Work out the finished part from the listing and answer in its coordinate system (mm). Face numbers are marked on the shaded views. A direction names the side the tool comes from. Give positions to 0.01 mm unless a question says otherwise; leave off trailing zeros. Write each loop counter-clockwise with the first axis right and the second up, starting at its lowest first coordinate (ties: lowest second). Pieces come first, ordered by that corner, then holes. Notation, with made-up numbers: (-21.75, 14.25) -> (-17.75, 14.25) arc R25 ccw to (-17.75, 48.25) -> close; hole circle Ø1 at (61, 43.5). An arc over 180 degrees is marked (long way). Write item = value, one per line. Start each with the question number.
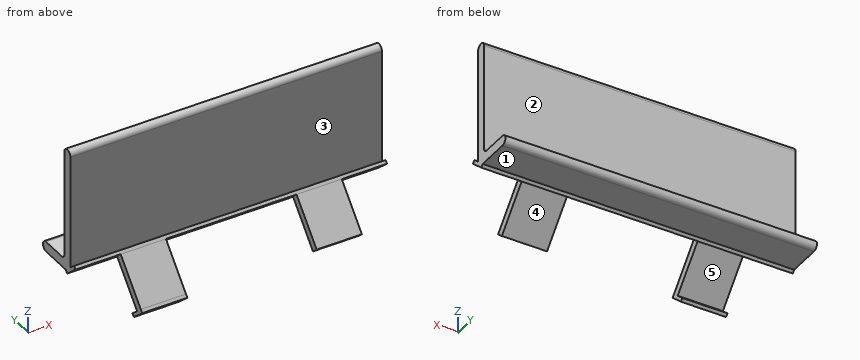
from build123d import *

# Parameters (mm, degrees)
F1_DEPTH = 155
F3_DEPTH = 155
F5_START = 22.5
F5_DEPTH = 22.5
F6_START = 110
F6_DEPTH = 22.5
F8_START = 22.5
F8_DEPTH = 22.5


# Not quite as in the source:
# - a feature of the source that left no trace in its solid (it failed there, or was rolled back) is left out


with BuildPart() as f1:
    # F0 (on Right) → F1 (new body)
    with BuildSketch(Plane.YZ):
        with BuildLine():
            Line((-25.3971134126, 39.5229434967), (-30.3971134126, 39.5229434967))
            Line((-30.3971134126, 39.5229434967), (-30.3971134126, -18.4770565033))
            ThreePointArc((-30.3971134126, -18.4770565033), (-29.811326975, -19.8912700657), (-28.3971134126, -20.4770565033))
            Line((-28.3971134126, -20.4770565033), (-10.3971134126, -20.4770565033))
            Line((-10.3971134126, -20.4770565033), (-10.3971134126, -15.4770565033))
            Line((-10.3971134126, -15.4770565033), (-23.3971134126, -15.4770565033))
            ThreePointArc((-23.3971134126, -15.4770565033), (-24.811326975, -14.8912700657), (-25.3971134126, -13.4770565033))
            Line((-25.3971134126, -13.4770565033), (-25.3971134126, 39.5229434967))
        make_face()
        with BuildLine():
            ThreePointArc((-25.3971134126, 39.5229434967), (-27.8971134126, 42.0229434967), (-30.3971134126, 39.5229434967))
            Line((-30.3971134126, 39.5229434967), (-25.3971134126, 39.5229434967))
        make_face()
        with BuildLine():
            Line((-10.3971134126, -15.4770565033), (-10.3971134126, -20.4770565033))
            ThreePointArc((-10.3971134126, -20.4770565033), (-7.8971134126, -17.9770565033), (-10.3971134126, -15.4770565033))
        make_face()
    extrude(amount=F1_DEPTH)

    # F2 (on Right) → F3 (join)
    with BuildSketch(Plane.YZ):
        Polygon((-26.6438154831, -20.4771793517), (-33.4096477321, -14.5422392527), (-34.530691973, -15.8202297886), (-27.764859724, -21.7551698876), align=None)
    extrude(amount=F3_DEPTH)

    # F4 (on Right) → F5 (join)
    with BuildSketch(Plane.YZ.offset(F5_START)):
        Polygon((-31.5236554179, -18.4579809437), (-34.530691973, -15.8202297886), (-51.0166366924, -34.614208258), (-48.0096001373, -37.2519594131), align=None)
    extrude(amount=F5_DEPTH)

    # F4 (on Right) → F6 (join)
    with BuildSketch(Plane.YZ.offset(F6_START)):
        Polygon((-31.5236554179, -18.4579809437), (-34.530691973, -15.8202297886), (-51.0166366924, -34.614208258), (-48.0096001373, -37.2519594131), align=None)
    extrude(amount=F6_DEPTH)

    # F7 (on Right) → F8 (join)
    with BuildSketch(Plane.YZ.offset(F8_START)):
        Polygon((-51.0166366924, -34.614208258), (-52.136497942, -35.8932355375), (-45.370665693, -41.8281756365), (-44.2508044434, -40.549148357), align=None)
    extrude(amount=F8_DEPTH)


solid = f1.part
(1) For the marked faces 1 and 2, determine the directions among +Z, -Z, +X, -X, +Y, -Y from which every point of the face is accessible in a straight line to the end or side of a thin tool.
(2) A cutting plane is placed at C-C, the plane z = 2.5. Write down the section's boundary in (x, y), then the cut area to 3 significant figures.
(3) Determine the mould class of the marked faces 3, 4 and 5 for opening direction Z: pulls with the +Z half, pulls with the -Z half, needs draft (parallel to the pull), parting line crosses it, or undercut.
(4) A cutting plane is placed at A-A, the plane y = -41.5. Write down the section's boundary in (x, z).
(5) Each of these flat-tipped pins is pushed along its axis until it touches: pin 1 (15.5 mm diameter, centred on y = -44.5, z = -21.5, fed in from -X); pin 2 (1 mm diameter, centred on x = 30.5, z = 13.5, fed in from +Y); pin 3 (1 mm diameter, centred on x = 129.5, y = -34, fed in from -Z); pin 4 (12 mm diameter, centred on x = 75, y = -46, fed in from +Z). Where does it stop, or does it pass through?
(6) Find the intervals of material crossed by line 1 along X through (y, z) = (-48.5, -33); line 2 along Y through (x, z) = (82.5, 2); line 3 along Z through (x, y) = (148, -19), in increasing order.
Results list:
q1.face_1 = -Z, +X, -X, +Y
q1.face_2 = +Z, +X, -X, +Y
q2.outline = (0, -30.4) -> (155, -30.4) -> (155, -25.4) -> (0, -25.4) -> close
q2.area = 775 mm²
q3.face_3 = needs draft
q3.face_4 = pulls with the -Z half
q3.face_5 = undercut
q4.outline = (22.5, -29.83) -> (45, -29.83) -> (45, -23.77) -> (22.5, -23.77) -> close; (110, -29.83) -> (132.5, -29.83) -> (132.5, -23.77) -> (110, -23.77) -> close
q5.pin_1 = 22.5
q5.pin_2 = -25.4
q5.pin_3 = -21.85
q5.pin_4 = through
q6.line_1 = 22.5 to 45, 110 to 132.5
q6.line_2 = -30.4 to -25.4
q6.line_3 = -20.48 to -15.48
